Here's how the part is built. I have some questions about the finished solid (model axes, mm). A direction names the side the tool comes from. Round coordinates to 2 decimals unless told otherwise and drop trailing zeros. Write each loop counter-clockwise with the first axis right and the second up, starting at its lowest first coordinate (ties: lowest second). Pieces come first, ordered by that corner, then holes. Notation, with made-up numbers: (64.5, 81) -> (88.5, 81) arc R11 cw to (88.5, 86) -> close; hole circle Ø8 at (87, 3). An arc over 180 degrees is marked (long way). Answer as CSV lines item,"result".
from build123d import *

# Parameters (mm, degrees)
BOSS_EXTRUDE1_DEPTH = 11
SKETCH3_R           = 3
CUT_EXTRUDE1_DEPTH  = 50
SKETCH4_R           = 2
CUT_EXTRUDE2_DEPTH  = 10


with BuildPart() as part:
    # Sketch2 → Boss-Extrude1 (new body)
    with BuildSketch(Plane.XY):
        Polygon((0, 19), (-50, 19), (-50, -19), (0, -19), (0, -14), (-45, -14), (-45, 14), (0, 14), align=None)
    extrude(amount=BOSS_EXTRUDE1_DEPTH)

    # Sketch3 → Cut-Extrude1 (cut)
    with BuildSketch(Plane(origin=(0, 19, 0), x_dir=(1, 0, 0), z_dir=(0, 1, 0))):
        with Locations(Location((-6, -5.559501776, 0), (0, 0, 180))):
            Circle(SKETCH3_R)
    extrude(amount=-CUT_EXTRUDE1_DEPTH, mode=Mode.SUBTRACT)

    # Sketch4 → Cut-Extrude2 (cut)
    with BuildSketch(Plane(origin=(-45, 0, 0), x_dir=(0, 0, -1), z_dir=(1, 0, 0))):
        with Locations((-5.5, 9)):
            Circle(SKETCH4_R)
        with Locations((-5.5, -9)):
            Circle(SKETCH4_R)
    extrude(amount=-CUT_EXTRUDE2_DEPTH, mode=Mode.SUBTRACT)


solid = part.part
Item 1: If we mould it in two halves opening along X, with no side actions, what happens to faces 3 (the cylindrical face through (-47.465, 10.983, 5.76)), 4 (the cylindrical face through (-8.77, -16.47, 4.41)), 5 (the flat face through (-45, 0, 5))? For each: pulls with the +X half, pulls with the -X half, needs draft (parallel to the pull), parting line crosses it, or undercut.
Results found:
face 3,"needs draft"
face 4,"undercut"
face 5,"pulls with the +X half"
Item 2: Suppose I cut it at A-A, the plane x = -6. List the corners of the cut face in (y, z) for me.
Results found:
outline,"(-19, 0) -> (-14, 0) -> (-14, 2.56) -> (-19, 2.56) -> close; (-19, 8.56) -> (-14, 8.56) -> (-14, 11) -> (-19, 11) -> close; (14, 0) -> (19, 0) -> (19, 2.56) -> (14, 2.56) -> close; (14, 8.56) -> (19, 8.56) -> (19, 11) -> (14, 11) -> close"
Item 3: Will these pins go through, and if not, where does the flat tip stop? pin 1 (3.5 mm diameter, centred on y = 9, z = 5.5, fed in from -X); pin 2 (1.5 mm diameter, centred on y = 12.5, z = 2, fed in from +X).
Results found:
pin 1,"passes through"
pin 2,"stops at x = -45"
Item 4: Suppose I cut it at B-B, the plane z = 9.5. List the corners of the cut face in (x, y) for me, then the cut area to 3 significant figures.
Results found:
outline,"(-50, -19) -> (0, -19) -> (0, -14) -> (-45, -14) -> (-45, 14) -> (0, 14) -> (0, 19) -> (-50, 19) -> close"
area,"640 mm²"
Item 5: For faces 1 (the flat face through (-23, 14, 5)), 2 (the flat face through (-50, 0, 5)), which set-ups out of +Z, -Z, +X, -X, +Y, -Y let a thin tool reach every point of the face, with its end or its side?
Results found:
face 1,"+Z, -Z, +X"
face 2,"+Z, -Z, -X, +Y, -Y"
Item 6: Suppose I cut it at C-C, the plane y = 9. List the corners of the cut face in (x, z) for me, then the cut area to 3 significant figures.
Results found:
outline,"(-50, 0) -> (-45, 0) -> (-45, 3.5) -> (-50, 3.5) -> close; (-50, 7.5) -> (-45, 7.5) -> (-45, 11) -> (-50, 11) -> close"
area,"35.0 mm²"
Item 7: Suppose I cut it at D-D, the plane x = -12.5. List the corners of the cut face in (y, z) for me.
Results found:
outline,"(-19, 0) -> (-14, 0) -> (-14, 11) -> (-19, 11) -> close; (14, 0) -> (19, 0) -> (19, 11) -> (14, 11) -> close"
Item 8: I need wall thicknesses on L1, parallel to Y at x = -47.3, z = 5.5; L2, parallel to Y at x = -30, z = 9; L3, parallel to Z at x = -6, y = 17. Which ranges of each line are inside material? Lowest first, please.
Results found:
L1,"y = -19 to -11, -7 to 7, 11 to 19"
L2,"y = -19 to -14, 14 to 19"
L3,"z = 0 to 2.56, 8.56 to 11"
